Could you check a few things on this model? Use its own coordinates, in mm. A direction names the side the tool comes from. Coordinates: 2 decimals unless noted, no trailing zeros. Loops run counter-clockwise (first coordinate to the right, second up) from the corner with the lowest first, then second, coordinate; pieces in that order, holes last. Notation, with made-up numbers: (72, 51.25) -> (114, 51.25) arc R20 ccw to (114, 55.25) -> close; hole circle Ø4 at (32, 33). An arc over 180 degrees is marked (long way). One line per question, with ' | ' between items.
```python
from build123d import *

# Parameters (mm, degrees)
EXTRUDE1_DEPTH = 150
SKETCH3_W      = 300
SKETCH3_H      = 10
EXTRUDE2_DEPTH = 50
SKETCH4_W      = 300
SKETCH4_H      = 10
EXTRUDE3_DEPTH = 100
SKETCH5_W      = 50
SKETCH5_H      = 16.996037372
EXTRUDE4_DEPTH = 365.725924497
EXTRUDE5_DEPTH = 3
EXTRUDE6_START = -5
SKETCH7_R      = 2.5
EXTRUDE6_DEPTH = 5


with BuildPart() as part:
    # Sketch1 → Extrude1 (new, symmetric)
    with BuildSketch(Plane(origin=(0, 0, 0), x_dir=(0, 0, -1), z_dir=(1, 0, 0))):
        Polygon((15, 5), (100, 5), (100, -5), (-100, -5), (-100, 5), (-15, 5), (-15, 10), (-20, 10), (-20, 12), (20, 12), (20, 10), (15, 10), align=None)
    extrude(amount=EXTRUDE1_DEPTH, both=True)

    # Sketch3 → Extrude2 (add)
    with BuildSketch(Plane(origin=(0, 5, 0), x_dir=(1, 0, 0), z_dir=(0, 1, 0))):
        with Locations((0, 95)):
            Rectangle(SKETCH3_W, SKETCH3_H)
    extrude(amount=EXTRUDE2_DEPTH)

    # Sketch4 → Extrude3 (add)
    with BuildSketch(Plane(origin=(0, 0, -100), x_dir=(-1, 0, 0), z_dir=(0, 0, -1))):
        with Locations((0, 50)):
            Rectangle(SKETCH4_W, SKETCH4_H)
    extrude(amount=EXTRUDE3_DEPTH)

    # Sketch5 → Extrude4 (cut, through all)
    with BuildSketch(Plane(origin=(150, 0, 0), x_dir=(0, 0, -1), z_dir=(1, 0, 0))):
        with Locations((145, 58.784793496)):
            Rectangle(SKETCH5_W, SKETCH5_H)
    extrude(amount=-EXTRUDE4_DEPTH, mode=Mode.SUBTRACT)

    # Sketch6 → Extrude5 (add)
    with BuildSketch(Plane(origin=(0, 0, -170), x_dir=(-1, 0, 0), z_dir=(0, 0, -1))):
        with BuildLine():
            Line((30, 62), (32.5, 62))
            ThreePointArc((32.5, 62), (35, 64.5), (37.5, 62))
            Line((37.5, 62), (40, 62))
            Line((40, 62), (40, 45))
            Line((40, 45), (30, 45))
            Line((30, 45), (30, 62))
        make_face()
    extrude(amount=-EXTRUDE5_DEPTH)

    # Sketch7 → Extrude6 (add)
    with BuildSketch(Plane.XY.offset(-167).offset(EXTRUDE6_START)):
        with Locations((-35, 62)):
            Circle(SKETCH7_R)
    extrude(amount=EXTRUDE6_DEPTH)


solid = part.part
```
Q1. Please list where these lines run through material, in increasing order: L1, parallel to Z at x = -128.5, y = 9; L2, parallel to Z at x = -88.5, y = -2; L3, parallel to Z at x = -126, y = 47.5. Write a range as [from, to].
Values follow:
L1: z = [-100, -90], [-15, 15] | L2: z = [-100, 100] | L3: z = [-200, -90]
Q2. For faces 4 (the face through (-35, 56, -167)), 5 (the face through (2, 12, 0)), 6 (the face through (2, -5, -1)), 7 (the face through (2, 45, -149)), which set-ups out of +Z, -Z, +X, -X, +Y, -Y let a thin tool reach every point of the face, with its end or its side?
Values follow:
face 4: +X, -X, +Y | face 5: +Z, +X, -X, +Y | face 6: +Z, -Z, +X, -X, -Y | face 7: -Z, +X, -X, -Y
Q3. Imagine slicing it at C-C on y = 23.5. Write out the boundary of the cut face in (x, z), plus the area to 3 significant figures.
Values follow:
outline: (-150, -100) -> (150, -100) -> (150, -90) -> (-150, -90) -> close | area: 3,000 mm2
Q4. We'd pull the mould along Z, two halves only. Please class faces 1 (the face through (2, 5, 58)), 2 (the face through (2, 50.287, -145)), 3 (the face through (2, 50, -200)): released by +Z, released by -Z, zero draft, split by the parting line, or undercut.
Values follow:
face 1: zero draft | face 2: undercut | face 3: released by -Z
Q5. Imagine slicing it at A-A on x = 127.5. Write out the boundary of the cut face in (y, z).
Values follow:
outline: (-5, -100) -> (45, -100) -> (45, -200) -> (55, -200) -> (55, -170) -> (50.29, -170) -> (50.29, -120) -> (55, -120) -> (55, -90) -> (5, -90) -> (5, -15) -> (10, -15) -> (10, -20) -> (12, -20) -> (12, 20) -> (10, 20) -> (10, 15) -> (5, 15) -> (5, 100) -> (-5, 100) -> close
Q6. Imagine slicing it at B-B on z = -1.5. Write out the boundary of the cut face in (x, y), plus the area to 3 significant figures.
Values follow:
outline: (-150, -5) -> (150, -5) -> (150, 12) -> (-150, 12) -> close | area: 5,100 mm2
Q7. For pin 1 (2.5 mm diameter, centred on x = 65, y = 7, fed in from -Z); pin 2 (1.5 mm diameter, centred on x = 14.5, z = -166, fed in from +Y); pin 3 (4 mm diameter, centred on x = -44, y = 12.5, fed in from +Z), each with a flat end and sliding along its axis, tell me the tip position at first contact or that it passes through.
Values follow:
pin 1: stops at z = -100 | pin 2: stops at y = 50.29 | pin 3: stops at z = 20
